Geometry: final body of the model. Coordinates: model frame, mm. A direction names the side the tool comes from. Round coordinates to 2 decimals unless told otherwise and drop trailing zeros. Loops run counter-clockwise (first coordinate to the right, second up) from the corner with the lowest first, then second, coordinate; pieces in that order, holes last. Notation, with made-up numbers: (27, 68) -> (33, 68) arc R11 cw to (33, 72) -> close; hole circle Ø9 at (50.5, -23.75). An arc over 180 degrees is marked (long way). Answer in a Markdown table with one row per item.
```python
from build123d import *

# Parameters (mm, degrees)
SKETCH_1_W             = 800
SKETCH_1_H             = 400
EXTRUDE_1_DEPTH        = 20
CUT_EXTRUDE_1_DEPTH    = 4.2
FILLET_1_R             = 0.13
FILLET_2_R             = 0.7
CUT_EXTRUDE_2_DEPTH    = 895.650769854
HOLE_WIZARD_M6_1_D     = 5
HOLE_WIZARD_M6_1_DEPTH = 15
HOLE_WIZARD_M6_1_TIP   = 1.502151548


with BuildPart() as part:
    # 스케치1 → 보스-돌출1 (new body)
    with BuildSketch(Plane(origin=(0, 0, 0), x_dir=(1, 0, 0), z_dir=(0, 1, 0))):
        with Locations((400, 200)):
            Rectangle(SKETCH_1_W, SKETCH_1_H)
    extrude(amount=EXTRUDE_1_DEPTH)

    # 스케치2 → 컷-돌출1 (cut)
    with BuildSketch(Plane(origin=(0, 20, 0), x_dir=(1, 0, 0), z_dir=(0, 1, 0))):
        with BuildLine():
            Line((43.996963872, 379.05), (756.003036128, 379.05))
            ThreePointArc((756.003036128, 379.05), (771.592593786, 372.592593786), (778.05, 357.003036128))
            Line((778.05, 357.003036128), (778.05, 43.996963872))
            ThreePointArc((778.05, 43.996963872), (771.592593786, 28.407406214), (756.003036128, 21.95))
            Line((756.003036128, 21.95), (43.996963872, 21.95))
            ThreePointArc((43.996963872, 21.95), (28.407406214, 28.407406214), (21.95, 43.996963872))
            Line((21.95, 43.996963872), (21.95, 357.003036128))
            ThreePointArc((21.95, 357.003036128), (28.407406214, 372.592593786), (43.996963872, 379.05))
        make_face()
        with BuildLine():
            Line((43.996963872, 372.95), (756.003036128, 372.95))
            ThreePointArc((756.003036128, 372.95), (767.279242421, 368.279242421), (771.95, 357.003036128))
            Line((771.95, 357.003036128), (771.95, 43.996963872))
            ThreePointArc((771.95, 43.996963872), (767.279242421, 32.720757579), (756.003036128, 28.05))
            Line((756.003036128, 28.05), (43.996963872, 28.05))
            ThreePointArc((43.996963872, 28.05), (32.720757579, 32.720757579), (28.05, 43.996963872))
            Line((28.05, 43.996963872), (28.05, 357.003036128))
            ThreePointArc((28.05, 357.003036128), (32.720757579, 368.279242421), (43.996963872, 372.95))
        make_face(mode=Mode.SUBTRACT)
    extrude(amount=-CUT_EXTRUDE_1_DEPTH, mode=Mode.SUBTRACT)

    # 필렛1
    fillet_1_edges = [part.edges().sort_by_distance(p)[0] for p in [
        (28.407406214, 20, -372.592593786),
        (21.95, 20, -200.5),
        (28.407406214, 20, -28.407406214),
        (400, 20, -21.95),
        (771.592593786, 20, -28.407406214),
        (778.05, 20, -200.5),
        (771.592593786, 20, -372.592593786),
        (400, 20, -379.05),
        (32.720757579, 20, -368.279242421),
        (400, 20, -372.95),
        (767.279242421, 20, -368.279242421),
        (771.95, 20, -200.5),
        (767.279242421, 20, -32.720757579),
        (400, 20, -28.05),
        (32.720757579, 20, -32.720757579),
        (28.05, 20, -200.5),
    ]]
    fillet(fillet_1_edges, radius=FILLET_1_R)

    # 필렛2
    fillet_2_edges = [part.edges().sort_by_distance(p)[0] for p in [
        (28.407406214, 15.8, -372.592593786),
        (400, 15.8, -379.05),
        (771.592593786, 15.8, -372.592593786),
        (778.05, 15.8, -200.5),
        (771.592593786, 15.8, -28.407406214),
        (400, 15.8, -21.95),
        (28.407406214, 15.8, -28.407406214),
        (21.95, 15.8, -200.5),
        (400, 15.8, -372.95),
        (32.720757579, 15.8, -368.279242421),
        (28.05, 15.8, -200.5),
        (32.720757579, 15.8, -32.720757579),
        (400, 15.8, -28.05),
        (767.279242421, 15.8, -32.720757579),
        (771.95, 15.8, -200.5),
        (767.279242421, 15.8, -368.279242421),
    ]]
    fillet(fillet_2_edges, radius=FILLET_2_R)

    # 스케치3 → 컷-돌출2 (cut, through all)
    with BuildSketch(Plane(origin=(0, 20, 0), x_dir=(1, 0, 0), z_dir=(0, 1, 0))):
        with BuildLine():
            Line((45, 365), (755, 365))
            ThreePointArc((755, 365), (762.071067812, 362.071067812), (765, 355))
            Line((765, 355), (765, 45))
            ThreePointArc((765, 45), (762.071067812, 37.928932188), (755, 35))
            Line((755, 35), (45, 35))
            ThreePointArc((45, 35), (37.928932188, 37.928932188), (35, 45))
            Line((35, 45), (35, 355))
            ThreePointArc((35, 355), (37.928932188, 362.071067812), (45, 365))
        make_face()
    extrude(amount=-CUT_EXTRUDE_2_DEPTH, mode=Mode.SUBTRACT)

    # M6 나사 구멍1
    with Locations(Plane(origin=(0, 20, 0), x_dir=(1, 0, 0), z_dir=(0, 1, 0))):
        with Locations((10, 10), (10, 390), (790, 390), (790, 10), (400, 390), (400, 10)):
            Hole(HOLE_WIZARD_M6_1_D / 2, depth=HOLE_WIZARD_M6_1_DEPTH)
            with Locations((0, 0, -(HOLE_WIZARD_M6_1_DEPTH + HOLE_WIZARD_M6_1_TIP / 2))):  # 118° drill point
                Cone(0, HOLE_WIZARD_M6_1_D / 2, HOLE_WIZARD_M6_1_TIP, mode=Mode.SUBTRACT)


solid = part.part
```
Item 1: Cut plane A-A (x = 540). Output: boundary loops of the cut face in (y, z).
Answer:
| item | result |
|---|---|
| outline | (0, -400) -> (20, -400) -> (20, -379.18) arc R0.13 ccw to (19.87, -379.05) -> (16.5, -379.05) arc R0.7 cw to (15.8, -378.35) -> (15.8, -373.65) arc R0.7 cw to (16.5, -372.95) -> (19.87, -372.95) arc R0.13 ccw to (20, -372.82) -> (20, -365) -> (0, -365) -> close; (0, -35) -> (20, -35) -> (20, -28.18) arc R0.13 ccw to (19.87, -28.05) -> (16.5, -28.05) arc R0.7 cw to (15.8, -27.35) -> (15.8, -22.65) arc R0.7 cw to (16.5, -21.95) -> (19.87, -21.95) arc R0.13 ccw to (20, -21.82) -> (20, 0) -> (0, 0) -> close |
Item 2: Draft query along X for faces 4 (the face through (394, 10, 0)), 5 (the face through (32.845, 18.209, -32.597)), 6 (the face through (800, 10, -197)). Return one class per face: pulls with the +X half, pulls with the -X half, needs draft (parallel to the pull), parting line crosses it, or undercut.
Answer:
| item | result |
|---|---|
| face 4 | needs draft |
| face 5 | undercut |
| face 6 | pulls with the +X half |
Item 3: Cut plane C-C (y = 10.75). Output: boundary loops of the cut face in (x, z), then the cut area to 3 significant figures.
Answer:
| item | result |
|---|---|
| outline | (0, -400) -> (800, -400) -> (800, 0) -> (0, 0) -> close; hole circle Ø5 at (10, -390); hole circle Ø5 at (10, -10); hole (35, -355) arc R10 ccw to (45, -365) -> (755, -365) arc R10 ccw to (765, -355) -> (765, -45) arc R10 ccw to (755, -35) -> (45, -35) arc R10 ccw to (35, -45) -> close; hole circle Ø5 at (400, -390); hole circle Ø5 at (400, -10); hole circle Ø5 at (790, -390); hole circle Ø5 at (790, -10) |
| area | 79,100 mm² |
Item 4: Line query: probe 1 along Z at (x, y) = (790, 9.75); probe 2 along Z at (x, y) = (400, 12.25); probe 3 along Z at (x, y) = (255, 16.25). Output: solid intervals per line, ascending. Write a range as [from, to].
Answer:
| item | result |
|---|---|
| probe 1 | z = [-400, -392.5], [-387.5, -12.5], [-7.5, 0] |
| probe 2 | z = [-400, -392.5], [-387.5, -365], [-35, -12.5], [-7.5, 0] |
| probe 3 | z = [-400, -379], [-373, -365], [-35, -28], [-22, 0] |
Item 5: Cut plane B-B (z = -154.5). Output: boundary loops of the cut face in (x, y).
Answer:
| item | result |
|---|---|
| outline | (0, 0) -> (35, 0) -> (35, 20) -> (28.18, 20) arc R0.13 ccw to (28.05, 19.87) -> (28.05, 16.5) arc R0.7 cw to (27.35, 15.8) -> (22.65, 15.8) arc R0.7 cw to (21.95, 16.5) -> (21.95, 19.87) arc R0.13 ccw to (21.82, 20) -> (0, 20) -> close; (765, 0) -> (800, 0) -> (800, 20) -> (778.18, 20) arc R0.13 ccw to (778.05, 19.87) -> (778.05, 16.5) arc R0.7 cw to (777.35, 15.8) -> (772.65, 15.8) arc R0.7 cw to (771.95, 16.5) -> (771.95, 19.87) arc R0.13 ccw to (771.82, 20) -> (765, 20) -> close |
Item 6: Reachability of faces 1 (the face through (0, 10, -197)), 2 (the face through (395, 10, -365)), 3 (the face through (771.42, 18.209, -372.763)) from +Z, -Z, +X, -X, +Y, -Y: full face, straight path, thin tool, end or side. Return the list, or none.
Answer:
| item | result |
|---|---|
| face 1 | +Z, -Z, -X, +Y, -Y |
| face 2 | +Y, -Y |
| face 3 | +Y |
